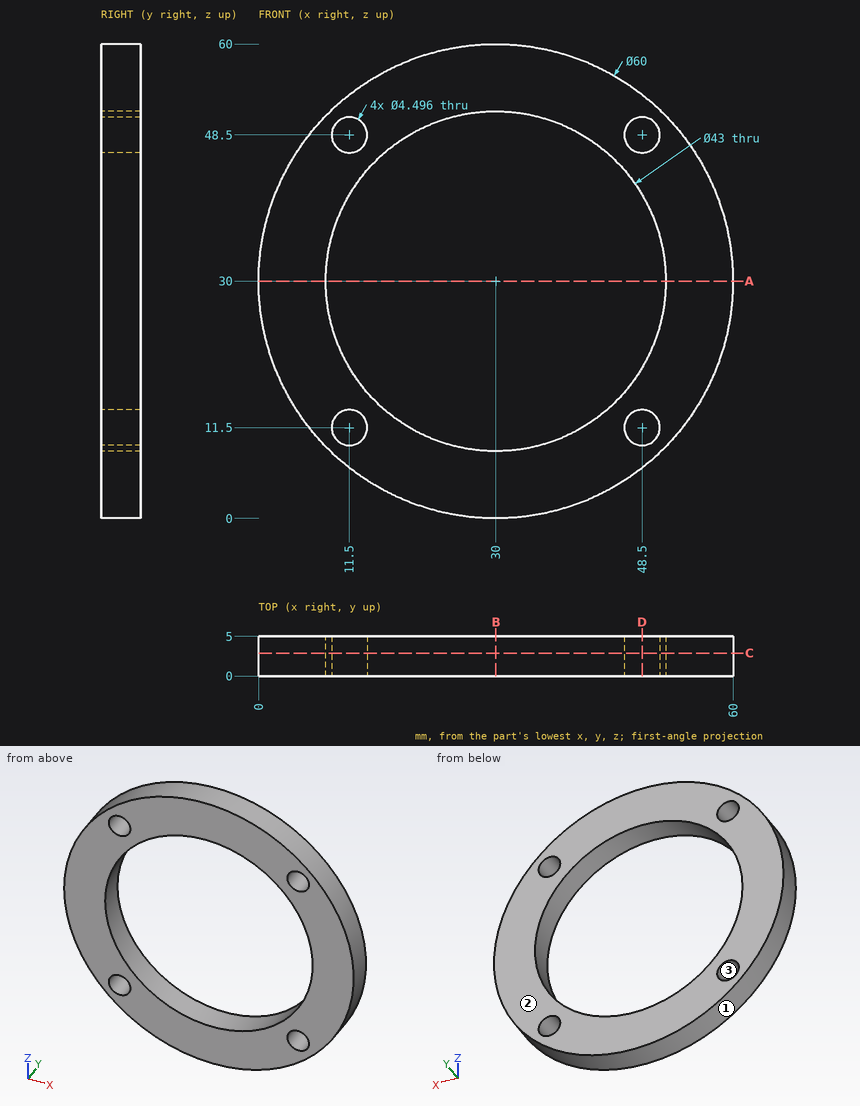
Geometry check sheet. Reference: drawing and pictorial views, mm from the part's lowest x, y, z. Round coordinates to 2 decimals unless told otherwise and drop trailing zeros. Order: outer loops, then holes, each group sorted by start corner. A loop starts at its lowest first (then second) coordinate and runs counter-clockwise, first axis right, second up. Notation, with made-up numbers: (86, 17) - (128, 17) arc R26 cw to (128, 53) - close; hole circle Ø7 at (7.5, -7). An arc over 180 degrees is marked (long way). Use a Markdown table: item, result. Add a question column.
1) Section check D-D (x = 48.5). Record the cut outline in (y, z), then the cut area to 3 significant figures.
2) Section check A-A (z = 30). Record the cut outline in (x, y), then the cut area to 3 significant figures.
3) Thickness scan on line 1 along Z through (x, y) = (30, 2.9); line 2 along X through (y, z) = (3.5, 11.5). Record the ranges inside material, lowest first.
4) Gauge pin test, flat ends, axial feed: P1, Ø1, axis at x = 48, y = 1, coming from the +Z side; P2, Ø2, axis at x = 38.5, y = 2.5, coming from the -Z side; P3, Ø1, axis at y = 4.5, z = 35.5, coming from the +X side. Record the tip position at first contact, or that the pin passes through.
5) Section check B-B (x = 30). Record the cut outline in (y, z), then the cut area to 3 significant figures.
6) Mould release check, pull along Z, two halves, no side actions. Record for the marked faces 1, 2 and 3: released by +Z, released by -Z, zero draft, split by the parting line, or undercut.
7) Section check C-C (y = 2.9). Record the cut outline in (x, z), then the cut area to 3 significant figures.
Established:
| question | item | result |
|---|---|---|
| 1 | outline | (0, 6.38) - (5, 6.38) - (5, 9.25) - (0, 9.25) - close; (0, 13.75) - (5, 13.75) - (5, 19.05) - (0, 19.05) - close; (0, 40.95) - (5, 40.95) - (5, 46.25) - (0, 46.25) - close; (0, 50.75) - (5, 50.75) - (5, 53.62) - (0, 53.62) - close |
| 1 | area | 81.7 mm2 |
| 2 | outline | (0, 0) - (8.5, 0) - (8.5, 5) - (0, 5) - close; (51.5, 0) - (60, 0) - (60, 5) - (51.5, 5) - close |
| 2 | area | 85.0 mm2 |
| 3 | line 1 | 0 to 8.5, 51.5 to 60 |
| 3 | line 2 | 6.38 to 9.25, 13.75 to 19.05, 40.95 to 46.25, 50.75 to 53.62 |
| 4 | P1 | z = 54.37 |
| 4 | P2 | z = 0.95 |
| 4 | P3 | x = 59.58 |
| 5 | outline | (0, 0) - (5, 0) - (5, 8.5) - (0, 8.5) - close; (0, 51.5) - (5, 51.5) - (5, 60) - (0, 60) - close |
| 5 | area | 85.0 mm2 |
| 6 | face 1 | split by the parting line |
| 6 | face 2 | zero draft |
| 6 | face 3 | undercut |
| 7 | outline | circle Ø60 at (30, 30); hole circle Ø43 at (30, 30); hole circle Ø4.5 at (11.5, 11.5); hole circle Ø4.5 at (11.5, 48.5); hole circle Ø4.5 at (48.5, 11.5); hole circle Ø4.5 at (48.5, 48.5) |
| 7 | area | 1,310 mm2 |
